Check sheet for the modelled part. Datum: model origin and axes. Units: mm. A direction names the side the tool comes from. Coordinates: 2 decimals unless noted, no trailing zeros. Loops run counter-clockwise (first coordinate to the right, second up) from the corner with the lowest first, then second, coordinate; pieces in that order, holes last. Notation, with made-up numbers: M -16.75,58.25 L 36.25,58.25 A14 cw 36.25,79.25 Z; hole C -24,-26 d4. An arc over 180 degrees is marked long. Return JSON: item names as keys, results as strings.
from build123d import *

# Parameters (mm, degrees)
EXTRUDE_1_DEPTH     = 1.2
EXTRUDE_START       = 1.2
SKETCH_1_3_R        = 3.5
EXTRUDE_2_DEPTH     = 8
SKETCH_2_R          = 2
CUT_EXTRUDE_1_DEPTH = 6


with BuildPart() as part:
    # Эскиз1 → Бобышка-Вытянуть1 (new body)
    with BuildSketch(Plane.XY):
        with BuildLine():
            Line((0, 22.5), (0, 3.5))
            ThreePointArc((0, 3.5), (1.025126266, 1.025126266), (3.5, 0))
            Line((3.5, 0), (82.5, 0))
            ThreePointArc((82.5, 0), (84.974873734, 1.025126266), (86, 3.5))
            Line((86, 3.5), (86, 22.5))
            ThreePointArc((86, 22.5), (84.974873734, 24.974873734), (82.5, 26))
            Line((82.5, 26), (3.5, 26))
            ThreePointArc((3.5, 26), (1.025126266, 24.974873734), (0, 22.5))
        make_face()
    extrude(amount=EXTRUDE_1_DEPTH)

    # Эскиз1<3> → Бобышка-Вытянуть2 (add)
    with BuildSketch(Plane.XY.offset(EXTRUDE_START)):
        with Locations((82.5, 22.5)):
            Circle(SKETCH_1_3_R)
        with Locations((82.5, 3.5)):
            Circle(SKETCH_1_3_R)
        with Locations((3.5, 22.5)):
            Circle(SKETCH_1_3_R)
        with Locations((3.5, 3.5)):
            Circle(SKETCH_1_3_R)
    extrude(amount=EXTRUDE_2_DEPTH)

    # Эскиз2 → Вырез-Вытянуть1 (cut)
    with BuildSketch(Plane.XY.offset(9.2)):
        with Locations((3.5, 22.5)):
            Circle(SKETCH_2_R)
        with Locations((3.5, 3.5)):
            Circle(SKETCH_2_R)
        with Locations((82.5, 22.5)):
            Circle(SKETCH_2_R)
        with Locations((82.5, 3.5)):
            Circle(SKETCH_2_R)
    extrude(amount=-CUT_EXTRUDE_1_DEPTH, mode=Mode.SUBTRACT)


solid = part.part
1) Section check B-B on y = 23.75. Record the cut outline in (x, z).
Answers:
{"outline": "M 0.23,0 L 85.77,0 L 85.77,9.2 L 84.06,9.2 L 84.06,3.2 L 80.94,3.2 L 80.94,9.2 L 79.23,9.2 L 79.23,1.2 L 6.77,1.2 L 6.77,9.2 L 5.06,9.2 L 5.06,3.2 L 1.94,3.2 L 1.94,9.2 L 0.23,9.2 Z"}
2) Set-up check for faces 1 (the face through (85, 4, 9.2)), 2 (the face through (84.408, 23.101, 6.242)): record each of +Z, -Z, +X, -X, +Y, -Y from which the full face is reachable in a straight line by a thin tool's end or side.
Answers:
{"face 1": "+Z, +X, -X, +Y, -Y", "face 2": "+Z"}
3) Section check A-A on z = 8. Record the cut outline in (x, y), then the cut area to 3 significant figures.
Answers:
{"outline": "C 3.5,3.5 d7; C 3.5,22.5 d7; C 82.5,3.5 d7; C 82.5,22.5 d7; hole C 3.5,3.5 d4; hole C 3.5,22.5 d4; hole C 82.5,3.5 d4; hole C 82.5,22.5 d4", "area": "104 mm²"}
4) Section check D-D on y = 4.25. Record the cut outline in (x, z).
Answers:
{"outline": "M 0,0 L 86,0 L 86,1.2 L 85.92,1.2 L 85.92,9.2 L 84.35,9.2 L 84.35,3.2 L 80.65,3.2 L 80.65,9.2 L 79.08,9.2 L 79.08,1.2 L 6.92,1.2 L 6.92,9.2 L 5.35,9.2 L 5.35,3.2 L 1.65,3.2 L 1.65,9.2 L 0.08,9.2 L 0.08,1.2 L 0,1.2 Z"}
5) Draft check along X on faces 3 (the face through (1.9, 21.3, 6.2)), 4 (the face through (42, 13, 0)). Enter one of: +X half, -X half, draft (parallel to the pull), parting line (faces both ways), or undercut.
Answers:
{"face 3": "undercut", "face 4": "draft"}
6) Go/stop test with flat-tipped pins: pin 1 Ø3.5 at (x, y) = (3.5, 3.5) entering from +Z; pin 2 Ø6 at (x, y) = (63.5, 4.5) entering from +Z. Record where each tip stops, or that it passes through.
Answers:
{"pin 1": "z = 3.2", "pin 2": "z = 1.2"}
7) Section check C-C on x = 71.5. Record the cut outline in (y, z), then the cut area to 3 significant figures.
Answers:
{"outline": "M 0,0 L 26,0 L 26,1.2 L 0,1.2 Z", "area": "31.2 mm²"}
8) Scan lines: line 1 along Y through (x, z) = (3.5, 5); line 2 along X through (y, z) = (21, 8); line 3 along Z through (x, y) = (13.5, 18.25). Record each from-to range of solid material in increasing order. Write a range as [from, to].
Answers:
{"line 1": "[0, 1.5], [5.5, 7], [19, 20.5], [24.5, 26]", "line 2": "[0.34, 2.18], [4.82, 6.66], [79.34, 81.18], [83.82, 85.66]", "line 3": "[0, 1.2]"}
